Here's how the part is built. I have some questions about the finished solid (model axes, mm). A direction names the side the tool comes from. Give positions to 0.01 mm unless a question says otherwise; leave off trailing zeros. Loops run counter-clockwise (first coordinate to the right, second up) from the corner with the lowest first, then second, coordinate; pieces in that order, holes last. Notation, with made-up numbers: (-34.75, 88) - (-25.75, 88) arc R24 cw to (-25.75, 127) - close; hole circle Ø3 at (2, -37). An arc over 180 degrees is marked (long way). Use one line per item in the form item = value.
from build123d import *

# Parameters (mm, degrees)
SM_BASE_FLANGE_1_DEPTH = 2
FILLET_1_R             = 3
CUT_EXTRUDE_1_DEPTH    = 10


# Sheet-metal steps are written as plain solids
with BuildPart() as part:
    # Sketch 1 → 基体-法兰1 (new body)
    with BuildSketch(Plane(origin=(0, 0, 0), x_dir=(1, 0, 0), z_dir=(0, 1, 0))):
        Polygon((-10, 7.5), (-18.5, 7.5), (-18.5, -7.5), (18.5, -7.5), (18.5, 7.5), (10, 7.5), (10, 16.146039932), (-10, 16.146039932), align=None)
    extrude(amount=-SM_BASE_FLANGE_1_DEPTH)

    # 圆角1
    fillet_1_edges = [part.edges().sort_by_distance(p)[0] for p in [
        (18.5, -1, -7.5),
        (18.5, -1, 7.5),
        (-18.5, -1, 7.5),
        (-18.5, -1, -7.5),
        (-10, -1, -7.5),
        (10, -1, -7.5),
    ]]
    fillet(fillet_1_edges, radius=FILLET_1_R)

    # 草图6 → 切除-拉伸1 (cut)
    with BuildSketch(Plane.XZ.offset(2)):
        with BuildLine():
            Line((-10.75, 4), (-10.75, -4))
            ThreePointArc((-10.75, -4), (-12.5, -5.75), (-14.25, -4))
            Line((-14.25, -4), (-14.25, 4))
            ThreePointArc((-14.25, 4), (-12.5, 5.75), (-10.75, 4))
        make_face()
        with BuildLine():
            Line((14.25, 4), (14.25, -4))
            ThreePointArc((14.25, -4), (12.5, -5.75), (10.75, -4))
            Line((10.75, -4), (10.75, 4))
            ThreePointArc((10.75, 4), (12.5, 5.75), (14.25, 4))
        make_face()
    extrude(amount=-CUT_EXTRUDE_1_DEPTH, mode=Mode.SUBTRACT)


solid = part.part
(1) For faces 1 (the flat face through (0, -1, 7.5)), 2 (the flat face through (10, -1, -13)), 3 (the cylindrical face through (-12.54, -1.01, 5.75)), which set-ups out of +Z, -Z, +X, -X, +Y, -Y let a thin tool reach every point of the face, with its end or its side?
Geometry says:
face_1 = +Z, +X, -X, +Y, -Y
face_2 = -Z, +X, +Y, -Y
face_3 = +Y, -Y
(2) If we section it at D-D (z = -12.75): List the corners of the cut face in (x, y) for me.
Geometry says:
outline = (-10, -2) - (10, -2) - (10, 0) - (-10, 0) - close
(3) If we section it at C-C (x = 12.5): List the corners of the cut face in (y, z) for me.
Geometry says:
outline = (-2, -7.54) - (0, -7.54) - (0, -5.75) - (-2, -5.75) - close; (-2, 5.75) - (0, 5.75) - (0, 7.5) - (-2, 7.5) - close
(4) If we section it at A-A (z = 2.5): List the corners of the cut face in (x, y) for me, plus the area to 3 significant figures.
Geometry says:
outline = (-18.5, -2) - (-14.25, -2) - (-14.25, 0) - (-18.5, 0) - close; (-10.75, -2) - (10.75, -2) - (10.75, 0) - (-10.75, 0) - close; (14.25, -2) - (18.5, -2) - (18.5, 0) - (14.25, 0) - close
area = 60.0 mm²
(5) Thinking about a two-plate mould opening in X: for faces 4 (the flat face through (-10, -1, -13)), 5 (the flat face through (14.25, -1, 0)), 6 (the flat face through (0, 0, -4)), which applies, pulls with the +X half, pulls with the -X half, needs draft (parallel to the pull), parting line crosses it, or undercut?
Geometry says:
face_4 = pulls with the -X half
face_5 = undercut
face_6 = needs draft
(6) If I drill on probe 1 along X at (y, z) = (-0.7, -0.5); probe 2 along X at (y, z) = (-0.4, -5.5); probe 3 along Z at (x, y) = (-15, -1.05), over which ranges is the centre line in solid material (lowest first)?
Geometry says:
probe_1 = -18.5 to -14.25, -10.75 to 10.75, 14.25 to 18.5
probe_2 = -18.33 to -13.4, -11.6 to 11.6, 13.4 to 18.33
probe_3 = -7.5 to 7.5
(7) If we section it at B-B (y = -1): List the corners of the cut face in (x, z) for me, plus the area to 3 significant figures.
Geometry says:
outline = (-18.5, -4.5) arc R3 ccw to (-15.5, -7.5) - (-13, -7.5) arc R3 cw to (-10, -10.5) - (-10, -16.15) - (10, -16.15) - (10, -10.5) arc R3 cw to (13, -7.5) - (15.5, -7.5) arc R3 ccw to (18.5, -4.5) - (18.5, 4.5) arc R3 ccw to (15.5, 7.5) - (-15.5, 7.5) arc R3 ccw to (-18.5, 4.5) - close; hole (-14.25, -4) arc R1.75 ccw to (-10.75, -4) - (-10.75, 4) arc R1.75 ccw to (-14.25, 4) - close; hole (10.75, -4) arc R1.75 ccw to (14.25, -4) - (14.25, 4) arc R1.75 ccw to (10.75, 4) - close
area = 649 mm²
(8) For P1, Ø1, axis at y = -1, z = -13, coming from the -X side; P2, Ø0.6, axis at x = -13.5, y = -1, coming from the -Z side, each with a flat end and sliding along its axis, tell me the tip position at first contact or that it passes through.
Geometry says:
P1 = -10
P2 = -7.5
